from build123d import *

# Parameters (mm, degrees)
MAIN_EXTRUSION_DEPTH = 25


with BuildPart() as part:
    # Sk Main Extrusion → Main Extrusion (new body)
    with BuildSketch(Plane.XY):
        with BuildLine():
            Line((-4.190076845, 16.671180212), (-5.222054351, 19.506515107))
            ThreePointArc((-5.222054351, 19.506515107), (-5.496641489, 19.864364033), (-5.926823816, 20))
            Line((-5.926823816, 20), (-18.5, 20))
            ThreePointArc((-18.5, 20), (-19.560660172, 19.560660172), (-20, 18.5))
            Line((-20, 18.5), (-20, 1.5))
            ThreePointArc((-20, 1.5), (-19.560660172, 0.439339828), (-18.5, 0))
            Line((-18.5, 0), (37.5, 0))
            ThreePointArc((37.5, 0), (38.560660172, 0.439339828), (39, 1.5))
            Line((39, 1.5), (39, 3.5))
            ThreePointArc((39, 3.5), (38.560660172, 4.560660172), (37.5, 5))
            Line((37.5, 5), (31.319331136, 5))
            ThreePointArc((31.319331136, 5), (31.252521542, 4.990907613), (31.190571617, 4.964291825))
            Line((31.190571617, 4.964291825), (30.378759519, 4.476505905))
            ThreePointArc((30.378759519, 4.476505905), (30.25, 4.44079773), (30.121240481, 4.476505905))
            Line((30.121240481, 4.476505905), (29.309428383, 4.964291825))
            ThreePointArc((29.309428383, 4.964291825), (29.247478458, 4.990907613), (29.180668864, 5))
            Line((29.180668864, 5), (23, 5))
            ThreePointArc((23, 5), (20.878679656, 5.878679656), (20, 8))
            Line((20, 8), (20, 18.5))
            ThreePointArc((20, 18.5), (19.560660172, 19.560660172), (18.5, 20))
            Line((18.5, 20), (5.926823816, 20))
            ThreePointArc((5.926823816, 20), (5.496641489, 19.864364033), (5.222054351, 19.506515107))
            Line((5.222054351, 19.506515107), (4.190076845, 16.671180212))
            ThreePointArc((4.190076845, 16.671180212), (4.175951325, 16.563886241), (4.208493649, 16.460675177))
            Line((4.208493649, 16.460675177), (4.987558066, 15.111296024))
            Line((4.987558066, 15.111296024), (5.718509166, 14.845251581))
            Line((5.718509166, 14.845251581), (8.396186179, 15.81984631))
            ThreePointArc((8.396186179, 15.81984631), (8.811074612, 15.786489799), (9.056960151, 15.450654467))
            ThreePointArc((9.056960151, 15.450654467), (8.933433013, 12.665882372), (7.504160339, 10.272684887))
            Line((7.504160339, 10.272684887), (6.540737726, 9.309262274))
            ThreePointArc((6.540737726, 9.309262274), (0, 6.6), (-6.540737726, 9.309262274))
            Line((-6.540737726, 9.309262274), (-7.504160339, 10.272684887))
            ThreePointArc((-7.504160339, 10.272684887), (-8.933433013, 12.665882372), (-9.056960151, 15.450654467))
            ThreePointArc((-9.056960151, 15.450654467), (-8.811074612, 15.786489799), (-8.396186179, 15.81984631))
            Line((-8.396186179, 15.81984631), (-5.718509166, 14.845251581))
            Line((-5.718509166, 14.845251581), (-4.987558066, 15.111296024))
            Line((-4.987558066, 15.111296024), (-4.208493649, 16.460675177))
            ThreePointArc((-4.208493649, 16.460675177), (-4.175951325, 16.563886241), (-4.190076845, 16.671180212))
        make_face()
        with BuildLine():
            Line((-9.797835979, 8.22371984), (-8.66205807, 7.08794193))
            ThreePointArc((-8.66205807, 7.08794193), (-7.88207258, 6.372610607), (-7.043254789, 5.727272727))
            ThreePointArc((-7.043254789, 5.727272727), (-6.475500267, 4.047732983), (-7.90569415, 3))
            Line((-7.90569415, 3), (-15.5, 3))
            ThreePointArc((-15.5, 3), (-16.560660172, 3.439339828), (-17, 4.5))
            Line((-17, 4.5), (-17, 15.5))
            ThreePointArc((-17, 15.5), (-16.560660172, 16.560660172), (-15.5, 17))
            Line((-15.5, 17), (-13.783837598, 17))
            ThreePointArc((-13.783837598, 17), (-12.666241809, 16.500489706), (-12.292980155, 15.334639535))
            ThreePointArc((-12.292980155, 15.334639535), (-11.855296302, 11.494998738), (-9.797835979, 8.22371984))
        make_face(mode=Mode.SUBTRACT)
        with BuildLine():
            Line((17, 15.5), (17, 4.5))
            ThreePointArc((17, 4.5), (16.560660172, 3.439339828), (15.5, 3))
            Line((15.5, 3), (7.90569415, 3))
            ThreePointArc((7.90569415, 3), (6.475500267, 4.047732983), (7.043254789, 5.727272727))
            ThreePointArc((7.043254789, 5.727272727), (7.88207258, 6.372610607), (8.66205807, 7.08794193))
            Line((8.66205807, 7.08794193), (9.797835979, 8.22371984))
            ThreePointArc((9.797835979, 8.22371984), (11.855296302, 11.494998738), (12.292980155, 15.334639535))
            ThreePointArc((12.292980155, 15.334639535), (12.666241809, 16.500489706), (13.783837598, 17))
            Line((13.783837598, 17), (15.5, 17))
            ThreePointArc((15.5, 17), (16.560660172, 16.560660172), (17, 15.5))
        make_face(mode=Mode.SUBTRACT)
    extrude(amount=-MAIN_EXTRUSION_DEPTH)


solid = part.part
Model file for the job. Use its own axes, mm. A direction names the side the tool comes from. Coordinates: 2 decimals unless noted, no trailing zeros. Write each loop counter-clockwise with the first axis right and the second up, starting at its lowest first coordinate (ties: lowest second). Pieces come first, ordered by that corner, then holes. Notation, with made-up numbers: (23.25, -12.5) -> (75.25, -12.5) arc R28 ccw to (75.25, 8.5) -> close; hole circle Ø10 at (54.5, -37.75). An arc over 180 degrees is marked (long way). One line per item, written item: value. Start each with the question number.
1) Slice it at B-B on y = 12. Write the cut outline in (x, z), then the cut area to 3 significant figures.
2) Probe probe 1 along X at (y, z) = (13.75, -3.75); probe 2 along X at (y, z) = (7.5, -1); probe 3 along X at (y, z) = (5.5, -9.5). List the from-to ranges inside material, lowest first.
3) Slice it at D-D on x = 21. Write the cut outline in (y, z).
4) Slice it at A-A on x = -11.5. Write the cut outline in (y, z).
5) Slice it at C-C on z = -2. Count the separate pieces of the cut face and the enclosed holes in it, then the cut area to 3 significant figures.
6) Flat gauge pins, fed straight in: pin 1 Ø5 at (x, z) = (24, -4) entering from +Y; pin 2 Ø3 at (y, z) = (15, -7) entering from +X; pin 3 Ø12 at (y, z) = (11.5, -15) entering from +X; pin 4 Ø8 at (x, y) = (27.5, 13.5) entering from -Z. Where does each tip first touch, or does it go through?
7) Which spindle directions (+Z, -Z, +X, -X, +Y, -Y) get a long thin tool onto all of the face, cutting with end or side? Do faces 1 (the face through (26, 5, -12)), 2 (the face through (-11.873, 11.547, -12.325)), 3 (the face through (-19.55, 19.57, -12.32)). Say none if no direction does.
8) Pull direction X, two halves, no side cores. Call faces 4 (the face through (-16.55, 3.43, -12.32)), 5 (the face through (20, 13, -12)), 6 (the face through (-20, 10, -12)): +X half, -X half, draft (parallel to the pull), parting line (faces both ways), or undercut.
Answers follow:
1. outline: (-20, -25) -> (-17, -25) -> (-17, 0) -> (-20, 0) -> close; (-12.02, -25) -> (-8.69, -25) -> (-8.69, 0) -> (-12.02, 0) -> close; (8.69, -25) -> (12.02, -25) -> (12.02, 0) -> (8.69, 0) -> close; (17, -25) -> (20, -25) -> (20, 0) -> (17, 0) -> close
1. area: 316 mm2
2. probe 1: -20 to -17, -12.32 to -9.15, 9.15 to 12.32, 17 to 20
2. probe 2: -20 to -17, -9.07 to -3.98, 3.98 to 9.07, 17 to 20.04
2. probe 3: -20 to -17, -6.79 to 6.79, 17 to 21.34
3. outline: (0, -25) -> (5.76, -25) -> (5.76, 0) -> (0, 0) -> close
4. outline: (0, -25) -> (3, -25) -> (3, 0) -> (0, 0) -> close; (10.63, -25) -> (20, -25) -> (20, 0) -> (10.63, 0) -> close
5. separate pieces: 1
5. enclosed holes: 2
5. area: 536 mm2
6. pin 1: y = 5.4
6. pin 2: x = 20
6. pin 3: x = 21.34
6. pin 4: through
7. face 1: +Z, -Z, +X, +Y
7. face 2: +Z, -Z
7. face 3: +Z, -Z, -X, +Y
8. face 4: undercut
8. face 5: +X half
8. face 6: -X half
